The drawing under review shows one solid part. Ordinate dimensions are in mm from its lowest x, y, z. A direction names the side the tool comes from. Round coordinates to 2 decimals unless told otherwise and drop trailing zeros. Write each loop counter-clockwise with the first axis right and the second up, starting at its lowest first coordinate (ties: lowest second). Pieces come first, ordered by that corner, then holes. Notation, with made-up numbers: M 37,-39.5 L 69,-39.5 A12 ccw 69,-16.5 Z; hole C 71,31 d5. An arc over 180 degrees is marked long. One line per item, written item: value. Start each with the question number.
1) Take a section at A-A, the plane y = 12.5. Write out the cut boundary in (x, z).
2) Tool access review of the marked faces 1, 2 and 3: name each direction out of +Z, -Z, +X, -X, +Y, -Y from which nothing blocks a thin tool from reaching the whole face with its end or side.
3) Take a section at C-C, the plane z = 1.25. Write out the cut boundary in (x, y).
4) Take a section at B-B, the plane x = 18.5. Write out the cut boundary in (y, z), and give its area (3 significant figures).
5) Wall thickness on probe 1 along Y at (x, z) = (12.5, 8.75); probe 2 along X at (y, z) = (16.75, 9); probe 3 along X at (y, z) = (2.5, 7.5): over which ranges is each line inside the solid? List them lowest first.
6) For P1, Ø2, axis at y = 4.5, z = 7.5, coming from the +X side; P2, Ø0.8, axis at x = 2.5, z = 7.5, coming from the -Y side; P3, Ø2.5, axis at y = 11.5, z = 5.5, coming from the -X side, all flat-tipped, find the tip position at first contact; note any pin that passes through.
7) Mouldability with a two-part tool opening along X and no side actions: class the marked faces 4, 5 and 6 as +X half, -X half, draft (parallel to the pull), parting line (faces both ways), or undercut.
8) Take a section at D-D, the plane x = 7.5. Write out the cut boundary in (y, z), and give its area (3 significant figures).
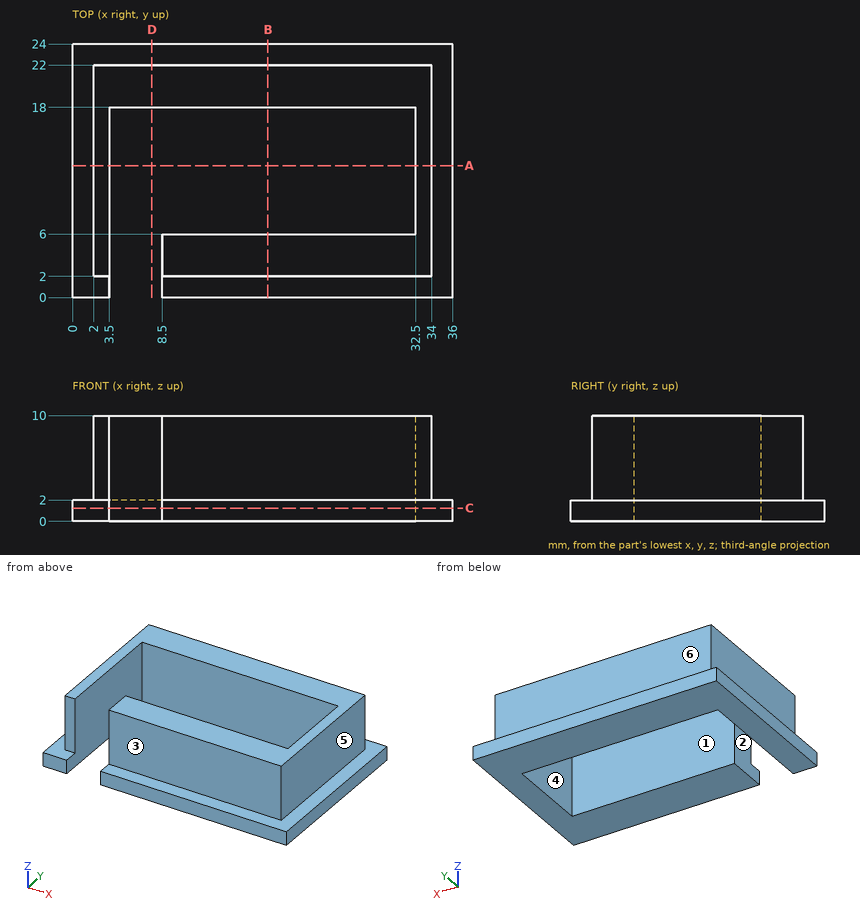
Checked values:
1. outline: M 0,0 L 3.5,0 L 3.5,10 L 2,10 L 2,2 L 0,2 Z; M 32.5,0 L 36,0 L 36,2 L 34,2 L 34,10 L 32.5,10 Z
2. face 1: +Z, -Z
2. face 2: +Z, -Z, -Y
2. face 3: +Z, +X, -X, -Y
3. outline: M 0,0 L 3.5,0 L 3.5,18 L 32.5,18 L 32.5,6 L 8.5,6 L 8.5,0 L 36,0 L 36,24 L 0,24 Z
4. outline: M 0,0 L 6,0 L 6,10 L 2,10 L 2,2 L 0,2 Z; M 18,0 L 24,0 L 24,2 L 22,2 L 22,10 L 18,10 Z
4. area: 88.0 mm2
5. probe 1: y = 2 to 6, 18 to 22
5. probe 2: x = 2 to 3.5, 32.5 to 34
5. probe 3: x = 2 to 3.5, 8.5 to 34
6. P1: stops at x = 34
6. P2: stops at y = 2
6. P3: stops at x = 2
7. face 4: undercut
7. face 5: +X half
7. face 6: draft
8. outline: M 18,0 L 24,0 L 24,2 L 22,2 L 22,10 L 18,10 Z
8. area: 44.0 mm2
